Source: three-view drawing plus pictorial views. Frame: mm from the lowest corner of the part. A direction names the side the tool comes from. Give positions to 0.01 mm unless a question says otherwise; leave off trailing zeros. Order: outer loops, then holes, each group sorted by start corner. A loop starts at its lowest first (then second) coordinate and runs counter-clockwise, first axis right, second up. Notation, with made-up numbers: M 24,70.25 L 70,70.25 A15 ccw 70,91.25 Z; hole C -7.5,40 d4. An arc over 180 degrees is marked long. One line per question, with ' | ' between items. Start each with the question number.
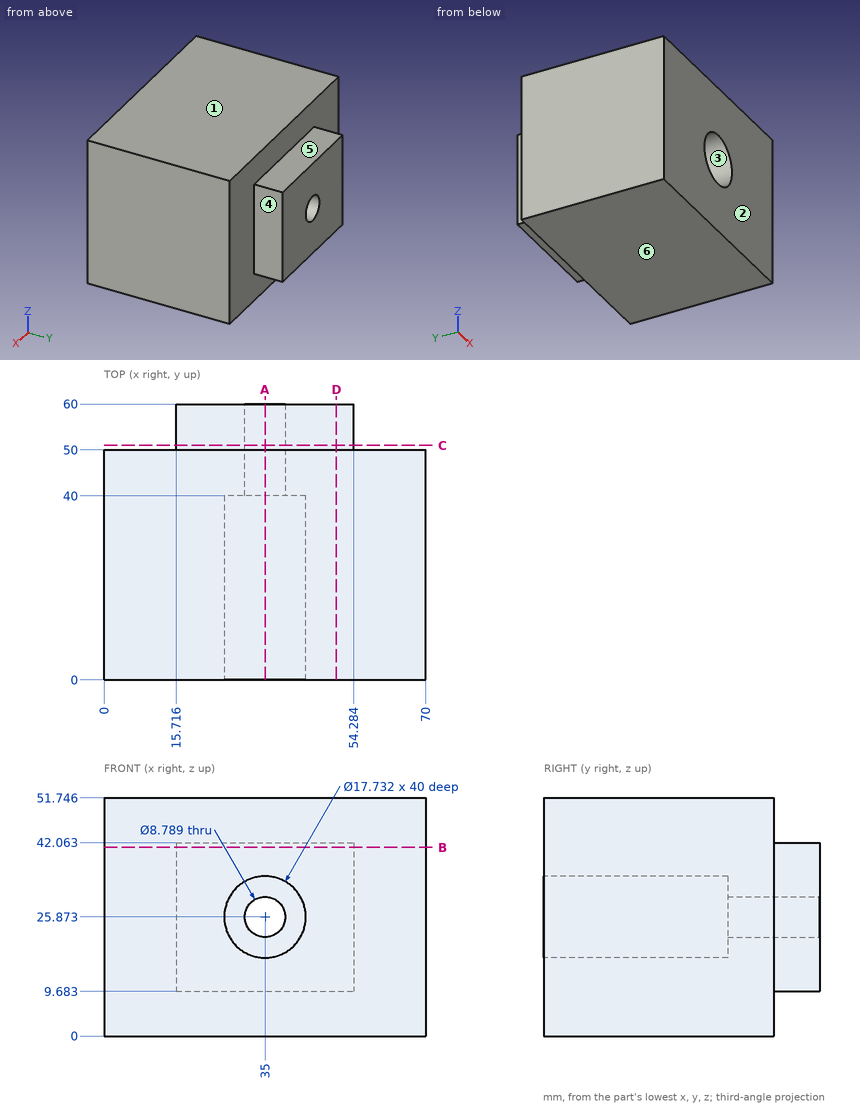
Item 1: Cut plane A-A on x = 35. Return the cut outline in (y, z), and give its area (3 significant figures).
Item 2: Reachability of the marked faces 4, 5 and 6 from +Z, -Z, +X, -X, +Y, -Y: full face, straight path, thin tool, end or side. Return the list, or none.
Item 3: Cut plane C-C on y = 51. Return the cut outline in (x, z) (1 decimal), and give its area (3 significant figures).
Item 4: Cut plane B-B on z = 41. Return the cut outline in (x, y) (1 decimal), and give its area (3 significant figures).
Item 5: Line query: line 1 (Z direction, x = 35, y = 15); line 2 (Y direction, x = 37, z = 3); line 3 (Y direction, x = 30.5, z = 23.5). Output: solid intervals per line, ascending.
Item 6: Cut plane D-D on x = 50.5. Return the cut outline in (y, z), and give its area (3 significant figures).
Item 7: Pin query (flat end, axial travel): pin 1 Ø14 at (x, z) = (35, 25.87) entering from -Y; pin 2 Ø11 at (x, y) = (41, 57.5) entering from +Z; pin 3 Ø8 at (y, z) = (57, 32.5) entering from +X. Return the tip coordinate at first contact, or that it passes through.
Item 8: Mould query, pull axis Z, two halves, no side actions, for the marked faces 1, 2 and 3. Classes: pulls with the +Z half, pulls with the -Z half, needs draft (parallel to the pull), parting line crosses it, or undercut.
Results are:
1) outline: M 0,0 L 50,0 L 50,9.68 L 60,9.68 L 60,21.48 L 40,21.48 L 40,17.01 L 0,17.01 Z; M 0,34.74 L 40,34.74 L 40,30.27 L 60,30.27 L 60,42.06 L 50,42.06 L 50,51.75 L 0,51.75 Z | area: 2,030 mm2
2) face 4: +Z, -Z, +X, +Y | face 5: +Z, +X, -X, +Y | face 6: -Z, +X, -X, +Y, -Y
3) outline: M 15.7,9.7 L 54.3,9.7 L 54.3,42.1 L 15.7,42.1 Z; hole C 35,25.9 d8.8 | area: 1,190 mm2
4) outline: M 0,0 L 70,0 L 70,50 L 54.3,50 L 54.3,60 L 15.7,60 L 15.7,50 L 0,50 Z | area: 3,890 mm2
5) line 1: z = 0 to 17.01, 34.74 to 51.75 | line 2: y = 0 to 50 | line 3: y = 40 to 60
6) outline: M 0,0 L 50,0 L 50,9.68 L 60,9.68 L 60,42.06 L 50,42.06 L 50,51.75 L 0,51.75 Z | area: 2,910 mm2
7) pin 1: stops at y = 40 | pin 2: stops at z = 42.06 | pin 3: stops at x = 54.28
8) face 1: pulls with the +Z half | face 2: needs draft | face 3: undercut
